The figure shows three views and two pictorial views of one solid part (mm, origin at its lowest corner). Answer the questions. A direction names the side the tool comes from. Give positions to 0.01 mm unless a question says otherwise; leave off trailing zeros. Order: outer loops, then holes, each group sorted by start corner. A loop starts at its lowest first (then second) coordinate and runs counter-clockwise, first axis right, second up. Notation, with made-up numbers: M 60.25,24.5 L 96.25,24.5 A27 cw 96.25,56.5 Z; hole C 55.5,27.25 d1. An arc over 180 degrees is marked long. One line per item, written item: value.
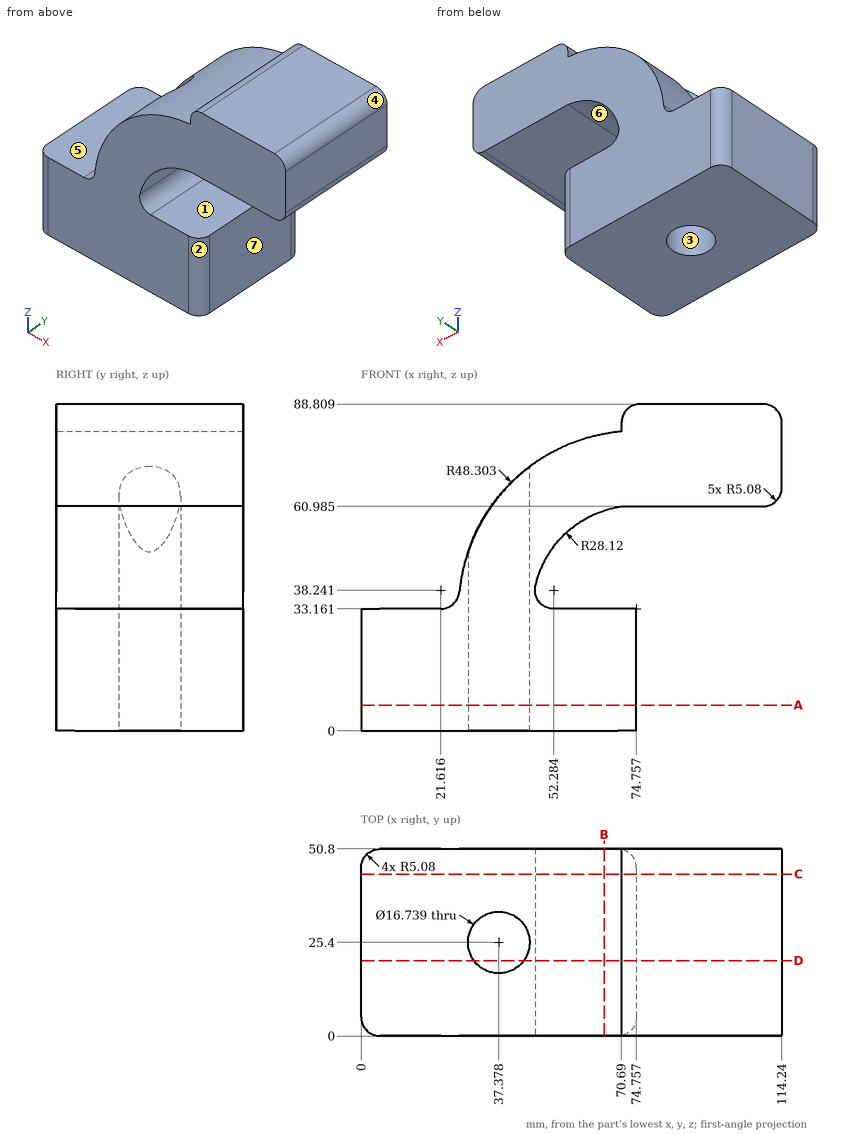
1) Determine the mould class of the marked faces 1, 2 and 3 for opening direction Y: +Y half, -Y half, draft (parallel to the pull), parting line (faces both ways), or undercut.
Reported:
face 1: draft
face 2: -Y half
face 3: undercut
2) Find section C-C, the plane y = 44. Write down the section's boundary in (x, z) (1 decimal), plus the area to 3 significant figures.
Reported:
outline: M 0,0 L 74.8,0 L 74.8,33.2 L 52.3,33.2 A5.1 cw 47.3,39.4 A28.1 cw 70.7,61 L 109.2,61 A5.1 ccw 114.2,66.1 L 114.2,83.7 A5.1 ccw 109.2,88.8 L 75.8,88.8 A5.1 ccw 70.7,83.7 L 70.7,81.3 A48.3 ccw 26.7,37.8 A5.1 cw 21.6,33.2 L 0,33.2 Z
area: 4,820 mm^2
3) Consider probe 1 along X at (y, z) = (25, 34) (1 decimal); probe 2 along X at (y, z) = (44, 26.5); probe 3 along Z at (x, y) = (73, 16.5) (1 decimal). Determine where each line is inside the solid, lowest interval first.
Reported:
probe 1: x = 24.4 to 29, 45.7 to 49.5
probe 2: x = 0 to 74.76
probe 3: z = 0 to 33.2, 61 to 88
4) Each of these flat-tipped pins is pushed along its axis until it touches: pin 1 Ø8 at (x, y) = (83, 21.5) entering from -Z (1 decimal); pin 2 Ø11 at (x, y) = (68, 13) entering from +Z (1 decimal); pin 3 Ø1.9 at (y, z) = (28, 83) entering from -X. Where does it stop, or does it pass through?
Reported:
pin 1: stops at z = 61
pin 2: stops at z = 88.3
pin 3: stops at x = 70.69
5) Find section A-A, the plane z = 7. Write down the section's boundary in (x, y).
Reported:
outline: M 0,5.08 A5.08 ccw 5.08,0 L 69.68,0 A5.08 ccw 74.76,5.08 L 74.76,45.72 A5.08 ccw 69.68,50.8 L 5.08,50.8 A5.08 ccw 0,45.72 Z; hole C 37.38,25.4 d16.74
6) Find section D-D, the plane y = 20.5. Write down the section's boundary in (x, z) (1 decimal), plus the area to 3 significant figures.
Reported:
outline: M 0,0 L 30.6,0 L 30.6,52.7 A48.3 ccw 26.7,37.8 A5.1 cw 21.6,33.2 L 0,33.2 Z; M 44.2,0 L 74.8,0 L 74.8,33.2 L 52.3,33.2 A5.1 cw 47.3,39.4 A28.1 cw 70.7,61 L 109.2,61 A5.1 ccw 114.2,66.1 L 114.2,83.7 A5.1 ccw 109.2,88.8 L 75.8,88.8 A5.1 ccw 70.7,83.7 L 70.7,81.3 A48.3 ccw 44.2,70.5 Z
area: 3,960 mm^2
7) Which of the six approach directions +Z, -Z, +X, -X, +Y, -Y give full straight-line access (tool end or side, diameter ignored) to the marked faces 4, 5, 6 and 7?
Reported:
face 4: +Z, +X, +Y, -Y
face 5: +Z, -X, +Y, -Y
face 6: +X, +Y, -Y
face 7: -Z, +X, +Y, -Y
8) Find section B-B, the plane x = 66. Write down the section's boundary in (y, z).
Reported:
outline: M 0,0 L 50.8,0 L 50.8,33.16 L 0,33.16 Z; M 0,59.88 L 50.8,59.88 L 50.8,80.66 L 0,80.66 Z
